```python
from build123d import *

# Parameters (mm, degrees)
BOSS_EXTRUDE1_DEPTH = 43.434
SKETCH3_W           = 3.81
SKETCH3_H           = 46.482
BOSS_EXTRUDE2_DEPTH = 43.688
BOSS_EXTRUDE5_DEPTH = 39.624
SKETCH9_R           = 6.35
CUT_EXTRUDE1_DEPTH  = 44.434
SKETCH10_R          = 1.5875
CUT_EXTRUDE2_DEPTH  = 4.81
SKETCH12_W          = 45.72
SKETCH12_H          = 43.434
BOSS_EXTRUDE6_DEPTH = 12.7
SKETCH13_W          = 45.72
SKETCH13_H          = 43.434
BOSS_EXTRUDE7_DEPTH = 12.7
SKETCH14_R          = 4.064
CUT_EXTRUDE3_DEPTH  = 6.35


with BuildPart() as part:
    # Sketch2 → Boss-Extrude1 (new body)
    with BuildSketch(Plane.XY.offset(816.492372385)):
        with BuildLine():
            Line((35.750095932, 34.097582937), (35.750095932, 33.285263123))
            ThreePointArc((35.750095932, 33.285263123), (35.457981836, 31.445408446), (34.772439624, 29.71323416))
            ThreePointArc((34.772439624, 29.71323416), (34.62798184, 28.864383796), (35.01595222, 28.095687512))
            Line((35.01595222, 28.095687512), (38.55890274, 24.552736992))
            ThreePointArc((38.55890274, 24.552736992), (39.005633691, 24.254240914), (39.532588778, 24.14942303))
            Line((39.532588778, 24.14942303), (43.443796213, 24.14942303))
            Line((43.443796213, 24.14942303), (43.443796213, 28.31442303))
            ThreePointArc((43.443796213, 28.31442303), (43.703006711, 28.940212531), (44.328796213, 29.19942303))
            Line((44.328796213, 29.19942303), (48.113296213, 29.19942303))
            Line((48.113296213, 29.19942303), (50.653296213, 29.19942303))
            Line((50.653296213, 29.19942303), (50.653296213, 10.45042303))
            Line((50.653296213, 10.45042303), (52.685296213, 10.45042303))
            Line((52.685296213, 10.45042303), (52.685296213, 56.93242303))
            Line((52.685296213, 56.93242303), (50.653296213, 56.93242303))
            Line((50.653296213, 56.93242303), (50.653296213, 38.18342303))
            Line((50.653296213, 38.18342303), (48.113296213, 38.18342303))
            Line((48.113296213, 38.18342303), (44.328796213, 38.18342303))
            ThreePointArc((44.328796213, 38.18342303), (43.703006711, 38.442633529), (43.443796213, 39.06842303))
            Line((43.443796213, 39.06842303), (43.443796213, 43.23342303))
            Line((43.443796213, 43.23342303), (39.532588778, 43.23342303))
            ThreePointArc((39.532588778, 43.23342303), (39.005633691, 43.128605146), (38.55890274, 42.830109068))
            Line((38.55890274, 42.830109068), (35.01595222, 39.287158548))
            ThreePointArc((35.01595222, 39.287158548), (34.62798184, 38.518462264), (34.772439624, 37.6696119))
            ThreePointArc((34.772439624, 37.6696119), (35.457981836, 35.937437615), (35.750095932, 34.097582937))
        make_face()
    extrude(amount=BOSS_EXTRUDE1_DEPTH)

    # Sketch3 → Boss-Extrude2 (add)
    with BuildSketch(Plane(origin=(52.685296213, 0, 0), x_dir=(0, 0, -1), z_dir=(1, 0, 0))):
        with Locations((-858.021372385, 33.69142303)):
            Rectangle(SKETCH3_W, SKETCH3_H)
    extrude(amount=BOSS_EXTRUDE2_DEPTH)

    # Sketch8 → Boss-Extrude5 (add)
    with BuildSketch(Plane(origin=(0, 0, 856.116372385), x_dir=(-1, 0, 0), z_dir=(0, 0, -1))):
        Polygon((-96.373296213, 56.93242303), (-52.685296213, 56.93242303), (-52.685296213, 54.90042303), (-94.087296213, 54.90042303), (-94.087296213, 42.220354744), (-96.373296213, 42.220354744), (-96.373296213, 54.90042303), align=None)
        Polygon((-96.373296213, 10.45042303), (-52.685296213, 10.45042303), (-52.685296213, 12.48242303), (-94.087296213, 12.48242303), (-94.087296213, 25.69042303), (-96.373296213, 25.69042303), (-96.373296213, 12.48242303), align=None)
    extrude(amount=BOSS_EXTRUDE5_DEPTH)

    # Sketch9 → Cut-Extrude1 (cut, through all)
    with BuildSketch(Plane.XY.offset(859.926372385)):
        with Locations((73.163747061, 34.125316724)):
            Circle(SKETCH9_R)
    extrude(amount=-CUT_EXTRUDE1_DEPTH, mode=Mode.SUBTRACT)

    # Sketch10 → Cut-Extrude2 (cut, through all)
    with BuildSketch(Plane(origin=(0, 0, 856.116372385), x_dir=(-1, 0, 0), z_dir=(0, 0, -1))):
        with Locations((-89.163747266, 50.124873673)):
            Circle(SKETCH10_R)
        with Locations((-57.921747266, 50.14642303)):
            Circle(SKETCH10_R)
        with Locations((-57.163746856, 18.90442303)):
            Circle(SKETCH10_R)
        with Locations((-88.405746856, 18.882873673)):
            Circle(SKETCH10_R)
    extrude(amount=-CUT_EXTRUDE2_DEPTH, mode=Mode.SUBTRACT)

    # Sketch12 → Boss-Extrude6 (add)
    with BuildSketch(Plane(origin=(0, 56.93242303, 0), x_dir=(1, 0, 0), z_dir=(0, 1, 0))):
        with Locations((73.513296213, -838.209372385)):
            Rectangle(SKETCH12_W, SKETCH12_H)
    extrude(amount=BOSS_EXTRUDE6_DEPTH)

    # Sketch13 → Boss-Extrude7 (add)
    with BuildSketch(Plane.XZ.offset(-10.45042303)):
        with Locations((73.513296213, 838.209372385)):
            Rectangle(SKETCH13_W, SKETCH13_H)
    extrude(amount=BOSS_EXTRUDE7_DEPTH)

    # Sketch14 → Cut-Extrude3 (cut)
    with BuildSketch(Plane.XY.offset(859.926372385)):
        with Locations((73.163747061, 63.28242303)):
            Circle(SKETCH14_R)
        with Locations((73.163747061, 4.10042303)):
            Circle(SKETCH14_R)
    extrude(amount=-CUT_EXTRUDE3_DEPTH, mode=Mode.SUBTRACT)


solid = part.part
```
Could you check a few things on this model? Use its own coordinates, in mm. A direction names the side the tool comes from. Round coordinates to 2 decimals unless told otherwise and drop trailing zeros. Loops run counter-clockwise (first coordinate to the right, second up) from the corner with the lowest first, then second, coordinate; pieces in that order, holes last. Notation, with made-up numbers: M 67.5,37 L 78.5,37 A5 cw 78.5,42 Z; hole C -16.75,-9.75 d4. An arc over 180 degrees is marked long. Put each result on its own line as item: value.
Q1. I need wall thicknesses on probe 1 along X at (y, z) = (50, 857); probe 2 along Y at (x, z) = (55.5, 822); probe 3 along X at (y, z) = (40, 829). Which ranges of each line are inside material? Lowest first, please.
Check result:
probe 1: 50.65 to 56.34, 59.5 to 87.58, 90.75 to 96.37
probe 2: -2.25 to 12.48, 54.9 to 69.63
probe 3: 35.73 to 43.44, 50.65 to 52.69
Q2. Thinking about a two-plate mould opening in X: for faces 1 (the face through (52.685, 33, 836)), 2 (the face through (95, 42.22, 837)), 3 (the face through (34.626, 28.877, 837.905)), which applies, released by +X, released by -X, zero draft, split by the parting line, or undercut?
Check result:
face 1: undercut
face 2: zero draft
face 3: released by -X
Q3. Imagine slicing it at B-B (x = 76). Write out the boundary of the cut face in (y, z), then the cut area to 3 significant figures.
Check result:
outline: M -2.25,816.49 L 12.48,816.49 L 12.48,856.12 L 28.44,856.12 L 28.44,859.93 L 7.01,859.93 L 7.01,853.58 L 1.19,853.58 L 1.19,859.93 L -2.25,859.93 Z; M 39.81,856.12 L 54.9,856.12 L 54.9,816.49 L 69.63,816.49 L 69.63,859.93 L 66.19,859.93 L 66.19,853.58 L 60.37,853.58 L 60.37,859.93 L 39.81,859.93 Z
area: 1,320 mm2
Q4. Imagine slicing it at D-D (y = 22.5). Write out the boundary of the cut face in (x, z), then the cut area to 3 significant figures.
Check result:
outline: M 50.65,816.49 L 52.69,816.49 L 52.69,856.12 L 94.09,856.12 L 94.09,816.49 L 96.37,816.49 L 96.37,859.93 L 50.65,859.93 Z
area: 345 mm2
Q5. Imagine slicing it at A-A (y = 36). Write out the boundary of the cut face in (x, z), then the cut area to 3 significant figures.
Check result:
outline: M 35.44,816.49 L 52.69,816.49 L 52.69,856.12 L 67.1,856.12 L 67.1,859.93 L 35.44,859.93 Z; M 79.23,856.12 L 96.37,856.12 L 96.37,859.93 L 79.23,859.93 Z
area: 869 mm2
Q6. For pin 1 (0.6 mm diameter, centred on y = 34, z = 847.5, fed in from -X); pin 2 (2 mm diameter, centred on y = 41, z = 836, fed in from +X); pin 3 (3 mm diameter, centred on x = 41.5, z = 845, fed in from +Y), each with a flat end and sliding along its axis, tell me the tip position at first contact or that it passes through.
Check result:
pin 1: x = 35.74
pin 2: x = 52.69
pin 3: y = 43.23
Q7. On a 3-axis mill with a long thin cutter (end or side, diameter ignored), from which of +Z, -Z, +X, -X, +Y, -Y can I reach the whole of each face in a straight line? I mean faces 4 (the face through (50.653, 14, 838)), 5 (the face through (50.653, 54, 839)), 6 (the face through (95, 25.69, 837)). Say none if no direction works.
Check result:
face 4: +Z, -Z, -Y
face 5: +Z, -Z, +Y
face 6: -Z, +X
